The figure shows three views and two pictorial views of one solid part (mm, origin at its lowest corner). Answer the questions. Give positions to 0.01 mm unless a question says otherwise; leave off trailing zeros. Order: outer loops, then holes, each group sorted by start corner. A loop starts at its lowest first (then second) coordinate and runs counter-clockwise, first axis right, second up. Notation, with made-up numbers: (-30.5, 6) -> (-20.5, 6) arc R28 cw to (-20.5, 36) -> close; hole circle Ø6 at (-4.75, 72.5). An arc over 180 degrees is marked (long way). One line per item, written item: value. Start each with the question number.
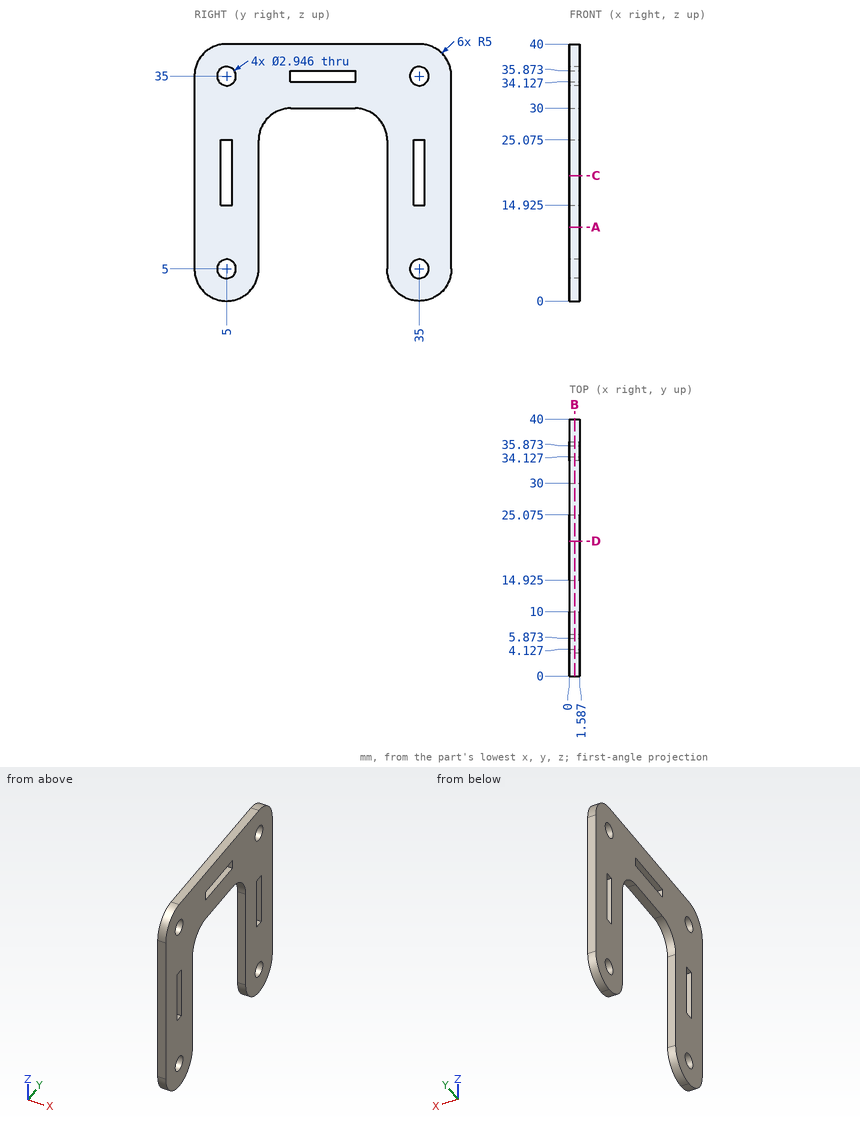
Item 1: Flat-ended cylindrical pins translate along their axes: pin 1 (8 mm diameter, centred on y = 16.5, z = 29.5, fed in from +X); pin 2 (2.5 mm diameter, centred on y = 35, z = 35, fed in from -X). Find the tip coordinate at first contact, or state that the pin passes through.
Item 2: Find section D-D on y = 21. Write down the section's boundary in (x, z).
Item 3: Find the intervals of material crossed by line 1 (Z direction, x = 0.7, y = 35) (1 decimal); line 2 (Y direction, x = 1.4, z = 16); line 3 (Z direction, x = 0.4, y = 15), in increasing order. Write a range as from..to.
Item 4: Find section C-C on z = 19.5. Write down the section's boundary in (x, y).
Item 5: Find section B-B on x = 0.8. Count the separate pieces of the cut face and the enclosed holes in it, then the cut area to 3 significant figures.
Item 6: Find section A-A on z = 11.5. Write down the section's boundary in (x, y).
Checks:
1. pin 1: x = 1.59
1. pin 2: through
2. outline: (0, 30) -> (1.59, 30) -> (1.59, 34.13) -> (0, 34.13) -> close; (0, 35.87) -> (1.59, 35.87) -> (1.59, 40) -> (0, 40) -> close
3. line 1: 0..3.5, 6.5..14.9, 25.1..33.5, 36.5..40
3. line 2: 0..4.13, 5.87..10, 30..34.13, 35.87..40
3. line 3: 30..34.13, 35.87..40
4. outline: (0, 0) -> (1.59, 0) -> (1.59, 4.13) -> (0, 4.13) -> close; (0, 5.87) -> (1.59, 5.87) -> (1.59, 10) -> (0, 10) -> close; (0, 30) -> (1.59, 30) -> (1.59, 34.13) -> (0, 34.13) -> close; (0, 35.87) -> (1.59, 35.87) -> (1.59, 40) -> (0, 40) -> close
5. separate pieces: 1
5. enclosed holes: 7
5. area: 898 mm2
6. outline: (0, 0) -> (1.59, 0) -> (1.59, 10) -> (0, 10) -> close; (0, 30) -> (1.59, 30) -> (1.59, 40) -> (0, 40) -> close
